from build123d import *

# Parameters (mm, degrees)
F0_W     = 50
F0_H     = 50
F1_DEPTH = 10
F2_W     = 8
F2_H     = 30
F3_DEPTH = 40
F4_R     = 14.99999
F6_D     = 5


# Not quite as in the source:
# - a fillet or chamfer is up to 0.001 mm smaller than in the source, because OpenCascade refuses the exact size


with BuildPart() as f1:
    # F0 (on Top) → F1 (new body)
    with BuildSketch(Plane.XY):
        with Locations((3.7194620818, 6.6150704944)):
            Rectangle(F0_W, F0_H)
    extrude(amount=F1_DEPTH)

    # F2 (on face) → F3 (join)
    with BuildSketch(Plane.XY.offset(10)):
        with Locations((-7.2805379182, 6.6150704944)):
            Rectangle(F2_W, F2_H)
        with Locations((14.7194620818, 6.6150704944)):
            Rectangle(F2_W, F2_H)
    extrude(amount=F3_DEPTH)

    # F4 (radius 15 in the source; OpenCascade refuses exactly that, so slightly less here)
    f4_edges = [f1.edges().sort_by_distance(p)[0] for p in [
        (-7.280538, -8.38493, 50),
        (-7.280538, 21.61507, 50),
        (14.719462, -8.38493, 50),
        (14.719462, 21.61507, 50),
    ]]
    fillet(f4_edges, radius=F4_R)

    # F6 (through all)
    with Locations(Plane.YZ.offset(18.7194620818)):
        with Locations((6.6150704944, 35)):
            Hole(F6_D / 2)


solid = f1.part
Check sheet for the modelled part. Datum: model origin and axes. Units: mm. A direction names the side the tool comes from. Coordinates: 2 decimals unless noted, no trailing zeros. Write each loop counter-clockwise with the first axis right and the second up, starting at its lowest first coordinate (ties: lowest second). Pieces come first, ordered by that corner, then holes.
Item 1: Access from +Z, -Z, +X, -X, +Y, -Y to the whole of each face (thin tool, end or side, straight path). Record for faces 1 (the face through (-3.281, 6, 30)), 2 (the face through (-7, -8.385, 22)), 3 (the face through (15, 21.615, 22)), 4 (the face through (18.719, 6, 30)).
Numbers:
face 1: +Z, +Y, -Y
face 2: +Z, +X, -X, -Y
face 3: +Z, +X, -X, +Y
face 4: +Z, +X, +Y, -Y
Item 2: Cross-section at A-A on z = 22. Record the boundary of the cut face in (x, y).
Numbers:
outline: (-11.28, -8.38) - (-3.28, -8.38) - (-3.28, 21.62) - (-11.28, 21.62) - close; (10.72, -8.38) - (18.72, -8.38) - (18.72, 21.62) - (10.72, 21.62) - close
Item 3: Mould release check, pull along X, two halves, no side actions. Record for faces 5 (the face through (3, -18.385, 5)), 6 (the face through (-11.281, 6, 30)), 7 (the face through (3, 7, 10)): released by +X, released by -X, zero draft, split by the parting line, or undercut.
Numbers:
face 5: zero draft
face 6: released by -X
face 7: undercut
Item 4: Scan lines: probe 1 along X at (y, z) = (-5, 24.5); probe 2 along Z at (x, y) = (6, -10.5); probe 3 along Y at (x, z) = (-5, 15). Record each from-to range of solid material in increasing order.
Numbers:
probe 1: x = -11.28 to -3.28, 10.72 to 18.72
probe 2: z = 0 to 10
probe 3: y = -8.38 to 21.62
Item 5: Cross-section at C-C on y = 14. Record the boundary of the cut face in (x, z).
Numbers:
outline: (-21.28, 0) - (28.72, 0) - (28.72, 10) - (18.72, 10) - (18.72, 48.06) - (10.72, 48.06) - (10.72, 10) - (-3.28, 10) - (-3.28, 48.06) - (-11.28, 48.06) - (-11.28, 10) - (-21.28, 10) - close
Item 6: Depth check by flat-ended pin: pin 1 Ø4 at (x, z) = (-7.5, 22) entering from -Y; pin 2 Ø8 at (y, z) = (6.62, 35) entering from -X; pin 3 Ø5 at (y, z) = (20, 14.5) entering from +X; pin 4 Ø12 at (y, z) = (3, 15.5) entering from +X. Enter the tip coordinate at first touch or a pass-through.
Numbers:
pin 1: stops at y = -8.38
pin 2: stops at x = -11.28
pin 3: stops at x = 18.72
pin 4: stops at x = 28.72
Item 7: Cross-section at D-D on x = -13.5. Record the boundary of the cut face in (y, z), then the cut area to 3 significant figures.
Numbers:
outline: (-18.38, 0) - (31.62, 0) - (31.62, 10) - (-18.38, 10) - close
area: 500 mm2
